from build123d import *

# Parameters (mm, degrees)
EXTRUDE_1_DEPTH = 6


with BuildPart() as part:
    # 草图1 → 凸台-拉伸1 (new body)
    with BuildSketch(Plane(origin=(0, 0, 0), x_dir=(1, 0, 0), z_dir=(0, 1, 0))):
        Polygon((30, 300), (24, 300), (24, 0), (30, 0), (30, -6), (80, -6), (80, 6), (130, 6), (130, -6), (180, -6), (180, 6), (230, 6), (230, -6), (280, -6), (280, 6), (380, 6), (380, -6), (430, -6), (430, 6), (480, 6), (480, -6), (530, -6), (530, 6), (580, 6), (580, -6), (630, -6), (630, 0), (636, 0), (636, 300), (630, 300), (630, 306), (580, 306), (580, 294), (530, 294), (530, 306), (480, 306), (480, 294), (430, 294), (430, 306), (380, 306), (380, 294), (280, 294), (280, 306), (230, 306), (230, 294), (180, 294), (180, 306), (130, 306), (130, 294), (80, 294), (80, 306), (30, 306), align=None)
        Polygon((340, 150), (340, 250), (540, 250), (540, 50), (340, 50), align=None, mode=Mode.SUBTRACT)
        Polygon((560, 150), (560, 275), (610, 275), (610, 25), (560, 25), align=None, mode=Mode.SUBTRACT)
        Polygon((100, 25), (100, 150), (100, 275), (50, 275), (50, 25), align=None, mode=Mode.SUBTRACT)
        Polygon((320, 50), (320, 150), (320, 250), (120, 250), (120, 50), align=None, mode=Mode.SUBTRACT)
    extrude(amount=EXTRUDE_1_DEPTH)


solid = part.part
Build history of the part. All positions in model axes, mm. Round coordinates to 2 decimals unless told otherwise and drop trailing zeros. Loops run counter-clockwise (first coordinate to the right, second up) from the corner with the lowest first, then second, coordinate; pieces in that order, holes last. Notation, with made-up numbers: (73, -14.75) -> (108, -14.75) arc R18 ccw to (108, 9.25) -> close; hole circle Ø1 at (-22.75, -36.5). An arc over 180 degrees is marked (long way). One line per item, written item: value. Start each with the question number.
Q1. Probe line 1 along X through (y, z) = (0.4, -205); line 2 along X through (y, z) = (3.55, -251); line 3 along Z through (x, y) = (353, 0.75). List the from-to ranges inside material, lowest first.
Q2. Cut at A-A on z = -137.5. List the corners of the cut face in (x, y), plus the area to 3 significant figures.
Q3. Cut at D-D on y = 4.55. Count the separate pieces of the cut face and the enclosed holes in it, plus the area to 3 significant figures.
Q4. Cut at B-B on x = 236.5. List the corners of the cut face in (y, z), plus the area to 3 significant figures.
Q5. Cut at C-C on z = -38. List the corners of the cut face in (x, y), plus the area to 3 significant figures.
Q6. Drop flat-ended pins along their axis: pin 1 Ø1.8 at (x, y) = (445, 4) entering from +Z; pin 2 Ø1.8 at (y, z) = (3, 2) entering from +X; pin 3 Ø3 at (y, z) = (3.5, 3) entering from -X. Give the stop position or say it passes through.
Computed:
1. line 1: 24 to 50, 100 to 120, 320 to 340, 540 to 560, 610 to 636
1. line 2: 24 to 50, 100 to 560, 610 to 636
1. line 3: -294 to -250, -50 to -6
2. outline: (24, 0) -> (50, 0) -> (50, 6) -> (24, 6) -> close; (100, 0) -> (120, 0) -> (120, 6) -> (100, 6) -> close; (320, 0) -> (340, 0) -> (340, 6) -> (320, 6) -> close; (540, 0) -> (560, 0) -> (560, 6) -> (540, 6) -> close; (610, 0) -> (636, 0) -> (636, 6) -> (610, 6) -> close
2. area: 672 mm²
3. separate pieces: 1
3. enclosed holes: 4
3. area: 78,600 mm²
4. outline: (0, -306) -> (6, -306) -> (6, -250) -> (0, -250) -> close; (0, -50) -> (6, -50) -> (6, 6) -> (0, 6) -> close
4. area: 672 mm²
5. outline: (24, 0) -> (50, 0) -> (50, 6) -> (24, 6) -> close; (100, 0) -> (560, 0) -> (560, 6) -> (100, 6) -> close; (610, 0) -> (636, 0) -> (636, 6) -> (610, 6) -> close
5. area: 3,070 mm²
6. pin 1: z = -6
6. pin 2: x = 630
6. pin 3: x = 30
